Can you work these out from the model? Positions are in its coordinate system, mm. Give positions to 0.01 mm unless a question says otherwise; leave off trailing zeros. Loops run counter-clockwise (first coordinate to the right, second up) from the corner with the lowest first, then second, coordinate; pieces in that order, holes last. Notation, with made-up numbers: (50.25, -32) - (86.25, -32) arc R15 cw to (86.25, -9) - close; hole circle Ø7 at (57, 68.25). An arc over 180 degrees is marked (long way). Answer in a Markdown table with one row per item.
from build123d import *

# Parameters (mm, degrees)
SKETCH1_W           = 203.2
SKETCH1_H           = 150
BOSS_EXTRUDE1_DEPTH = 1.5
FILLET1_R           = 12.7
SKETCH3_R           = 1.5
SKETCH3_W           = 15.875
SKETCH3_H           = 82.55
CUT_EXTRUDE2_DEPTH  = 127.319278022
CUT_EXTRUDE3_DEPTH  = 127.319278022
FILLET2_R           = 10


with BuildPart() as part:
    # Sketch1 → Boss-Extrude1 (new, symmetric)
    with BuildSketch(Plane(origin=(0, 0, 0), x_dir=(1, 0, 0), z_dir=(0, 1, 0))):
        Rectangle(SKETCH1_W, SKETCH1_H)
    extrude(amount=BOSS_EXTRUDE1_DEPTH, both=True)

    # Fillet1
    fillet1_edges = [part.edges().sort_by_distance(p)[0] for p in [
        (-101.6, 0, 75),
        (101.6, 0, 75),
        (101.6, 0, -75),
        (-101.6, 0, -75),
    ]]
    fillet(fillet1_edges, radius=FILLET1_R)

    # Sketch3 → Cut-Extrude2 (cut, through all)
    with BuildSketch(Plane.XZ.offset(1.5)):
        with Locations(Location((63.499999999, -62.3, 0), (0, 0, 270))):
            Circle(SKETCH3_R)
        with Locations(Location((73.024999999, 39.3, 0), (0, 0, 270))):
            Circle(SKETCH3_R)
        with Locations((79.25, -24.2)):
            Rectangle(SKETCH3_W, SKETCH3_H)
    cut_extrude2 = extrude(amount=-CUT_EXTRUDE2_DEPTH, mode=Mode.SUBTRACT)

    # Sketch4 → Cut-Extrude3 (cut, through all)
    with BuildSketch(Plane.XZ.offset(1.5)):
        with BuildLine():
            Line((101.6, 62.3), (101.6, 26.6))
            add(Edge.make_bspline(
                [(77.685809709, 75), (78.616134987, 72.645348103), (81.082482683, 67.616391475), (92.836364207, 54.857655975), (101.6, 41.84), (101.6, 26.6)],
                knots=[0.409925354, 0.409925354, 0.409925354, 0.409925354, 0.484619997, 0.584619997, 1, 1, 1, 1], degree=3))
            Line((77.685809709, 75), (88.9, 75))
            ThreePointArc((88.9, 75), (97.880256121, 71.280256121), (101.6, 62.3))
        make_face()
    cut_extrude3 = extrude(amount=-CUT_EXTRUDE3_DEPTH, mode=Mode.SUBTRACT)

    # Mirror1: Cut-Extrude2, Cut-Extrude3 across plane
    add(cut_extrude2.mirror(Plane(origin=(0, 0, 0), x_dir=(0, 0, 1), z_dir=(1, 0, 0))), mode=Mode.SUBTRACT)
    add(cut_extrude3.mirror(Plane(origin=(0, 0, 0), x_dir=(0, 0, 1), z_dir=(1, 0, 0))), mode=Mode.SUBTRACT)

    # Fillet2
    fillet2_edges = [part.edges().sort_by_distance(p)[0] for p in [
        (77.685809709, 0, 75),
        (-77.685809709, 0, 75),
    ]]
    fillet(fillet2_edges, radius=FILLET2_R)


solid = part.part
Q1. Imagine slicing it at B-B, the plane y = -1. Count the separate pieces of the cut face and the enclosed holes in it, and give its area (3 significant figures).
Checked values:
| item | result |
|---|---|
| separate pieces | 1 |
| enclosed holes | 6 |
| area | 26,900 mm² |
Q2. Imagine slicing it at A-A, the plane z = -27.5. Write out the boundary of the cut face in (x, y), and give its area (3 significant figures).
Checked values:
| item | result |
|---|---|
| outline | (-101.6, -1.5) - (-87.19, -1.5) - (-87.19, 1.5) - (-101.6, 1.5) - close; (-71.31, -1.5) - (71.31, -1.5) - (71.31, 1.5) - (-71.31, 1.5) - close; (87.19, -1.5) - (101.6, -1.5) - (101.6, 1.5) - (87.19, 1.5) - close |
| area | 514 mm² |
Q3. For pin 1 (2.5 mm diameter, centred on x = 73.025, z = 39.3, fed in from -Y); pin 2 (1 mm diameter, centred on x = -74, y = 1, fed in from +Z), each with a flat end and sliding along its axis, tell me the tip position at first contact or that it passes through.
Checked values:
| item | result |
|---|---|
| pin 1 | passes through |
| pin 2 | stops at z = 74.77 |
Q4. If I drill on line 1 (X direction, y = -0.05, z = -62.3); line 2 (X direction, y = -0.8, z = -17.5); line 3 (X direction, y = 0.1, z = 39.3) (3 decimals), over which ranges is the centre line in solid material (lowest first)? Write a range as [from, to].
Checked values:
| item | result |
|---|---|
| line 1 | x = [-101.6, -87.19], [-71.31, -65], [-62, 62], [65, 71.31], [87.19, 101.6] |
| line 2 | x = [-101.6, -87.19], [-71.31, 71.31], [87.19, 101.6] |
| line 3 | x = [-99.807, -74.525], [-71.525, 71.525], [74.525, 99.807] |
